Geometry check sheet. Reference: the model listing, model coordinates, mm. A direction names the side the tool comes from. Give positions to 0.01 mm unless a question says otherwise; leave off trailing zeros. Write each loop counter-clockwise with the first axis right and the second up, starting at its lowest first coordinate (ties: lowest second). Pieces come first, ordered by that corner, then holes. Notation, with made-up numbers: (36, 47) -> (88, 47) arc R3 cw to (88, 52) -> close; hole circle Ø9 at (26, 75.25). An arc over 180 degrees is marked (long way). One line per item, written item: value.
from build123d import *

# Parameters (mm, degrees)
F1_DEPTH = 177.8
F2_R     = 25.4
F3_DEPTH = 136.398
F4_R     = 25.4
F5_DEPTH = 138.684


with BuildPart() as f1:
    # F0 (on Right) → F1 (new body)
    with BuildSketch(Plane.YZ):
        Polygon((0, 0), (0, -88.9), (50.8, -88.9), (50.8, 114.3), (-50.8, 114.3), (-50.8, 25.4), align=None)
    extrude(amount=F1_DEPTH)

    # F2 (on Front) → F3 (cut)
    with BuildSketch(Plane.XZ):
        with Locations((50.8, 63.5)):
            Circle(F2_R)
        with Locations((127, -38.1)):
            Circle(F2_R)
    extrude(amount=-F3_DEPTH, mode=Mode.SUBTRACT)

    # F4 (on face) → F5 (cut)
    with BuildSketch(Plane(origin=(0, 50.8, 0), x_dir=(-1, 0, 0), z_dir=(0, 1, 0))):
        with Locations((-50.8, 63.5)):
            Circle(F4_R)
    extrude(amount=-F5_DEPTH, mode=Mode.SUBTRACT)


solid = f1.part
1) Tool access check on faces 1 (the flat face through (88, 1, 114.3)), 2 (the flat face through (88, 0, -44)). Record the directions out of +Z, -Z, +X, -X, +Y, -Y that give a thin tool (end or side, any length) a straight path to the whole face; none if there is none.
Verdict:
face 1: +Z, +X, -X, +Y, -Y
face 2: -Z, +X, -X, -Y
2) Mould release check, pull along Z, two halves, no side actions. Record for faces 3 (the cylindrical face through (151.227, 25.044, -30.471)), 4 (the flat face through (88, 25, -88.9)), 5 (the flat face through (177.8, 11, 37)): released by +Z, released by -Z, zero draft, split by the parting line, or undercut.
Verdict:
face 3: undercut
face 4: released by -Z
face 5: zero draft
3) Sectioned sample at C-C on y = 22.5. Record the cut outline in (x, z), plus the area to 3 significant figures.
Verdict:
outline: (0, -88.9) -> (177.8, -88.9) -> (177.8, 114.3) -> (0, 114.3) -> close; hole circle Ø50.8 at (50.8, 63.5); hole circle Ø50.8 at (127, -38.1)
area: 32,100 mm^2
4) Depth check by flat-ended pin: pin 1 Ø8 at (x, y) = (115.5, -30.5) entering from -Z; pin 2 Ø1.5 at (x, y) = (145.5, -13) entering from -Z (3 decimals). Enter the tip coordinate at first touch or a pass-through.
Verdict:
pin 1: z = 13.25
pin 2: z = 6.125
5) Sectioned sample at B-B on x = 127. Record the cut outline in (y, z).
Verdict:
outline: (-50.8, 25.4) -> (0, 0) -> (0, -12.7) -> (50.8, -12.7) -> (50.8, 114.3) -> (-50.8, 114.3) -> close; (0, -88.9) -> (50.8, -88.9) -> (50.8, -63.5) -> (0, -63.5) -> close
6) Sectioned sample at D-D on y = -11.5. Record the cut outline in (x, z), plus the area to 3 significant figures.
Verdict:
outline: (0, 5.75) -> (177.8, 5.75) -> (177.8, 114.3) -> (0, 114.3) -> close; hole circle Ø50.8 at (50.8, 63.5)
area: 17,300 mm^2
7) Sectioned sample at A-A on z = -38.1. Record the cut outline in (x, y).
Verdict:
outline: (0, 0) -> (101.6, 0) -> (101.6, 50.8) -> (0, 50.8) -> close; (152.4, 0) -> (177.8, 0) -> (177.8, 50.8) -> (152.4, 50.8) -> close
8) Scan lines: probe 1 along X at (y, z) = (37, -38); probe 2 along X at (y, z) = (-36.5, 63.5); probe 3 along Y at (x, z) = (62, -18). Record each from-to range of solid material in increasing order.
Verdict:
probe 1: 0 to 101.6, 152.4 to 177.8
probe 2: 0 to 25.4, 76.2 to 177.8
probe 3: 0 to 50.8
